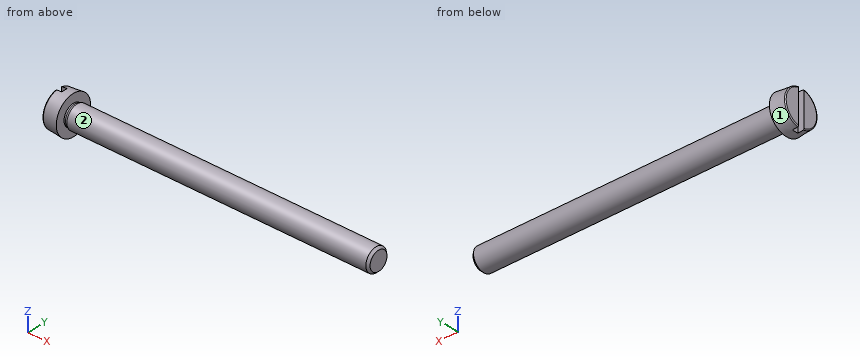
Autodesk Inventor part; units mm, degrees
ref_plane "Work Plane1" through (30.1625, 0, 0) normal (0, 0, -1) x (1, 0, 0)
ref_plane "YZ Plane" through (0, 0, 0) normal (1, 0, 0) x (0, 1, 0)
ref_plane "XZ Plane" through (0, 0, 0) normal (0, 1, 0) x (-1, 0, 0)
sketch "Skizze1" plane through (0, 0, 0) normal (0, 0, 1) x (1, 0, 0)
  line L0 (-3.9, 0) -> (80, 0)
  line L1 (80, 0) -> (80, 3)
  line L2 (80, 3) -> (1, 3)
  line L3 (1, 3) -> (0.3864, 2.7294)
  line L4 (0.3864, 2.7294) -> (0, 2.7294)
  line L5 (0, 2.7294) -> (0, 5)
  line L6 (-20.68, 0) -> (96.78, 0)
  line L7 (0, -1) -> (0, 6)
  line L8 (-3.9, 0) -> (-3.9, 4.6588)
  line L9 (0, 5) -> (-3.9, 4.6588)
  line L10 (1, 3) -> (0, 3) construction
  dimension "d0" = 80
  dimension "d1" = 79
  dimension "d2" = 0.6136
  dimension "d3" = 3.9
  dimension "d4" = 6
  dimension "d5" = 5.4587
  dimension "d9" = 10
  dimension "d10" = 5
revolve "Körper" add sketch "Skizze1" angle 360 about axis through (-3.9, 0, 0) along (1, 0, 0)
sketch "Skizze2" plane through (-3.9, 0, 0) normal (-1, 0, 0) x (0, 0, 1)
  circle A0 centre (0, 0) radius 5
  line L0 (0, 0) -> (0, 4.6588)
  line L1 (-5, 0.8) -> (5, 0.8)
  line L2 (5, 0.8) -> (5, -0.8)
  line L3 (5, -0.8) -> (-5, -0.8)
  line L4 (-5, -0.8) -> (-5, 0.8)
  line L5 (-5, 0) -> (5, 0) construction
  line L6 (0, 0.8) -> (0, -0.8) construction
  dimension "d11" = 1.6
  dimension "d12" = 10
fillet "Rundung1" radius 0.25 1 edges at (-3.9, -4.6588, 0)
extrude "Loch" cut sketch "Skizze2" against normal blind 1.6 contours A0 L3 L1 | L2 L3 A0 | A0 L1 L2 | A0 L4 L1 | L3 L4 A0
thread "Gewinde"
chamfer "Fase1" distance 0.5413 distance2 0.6136 1 edges at (80, -3, 0) measured on face at (80, 0.8631, 0.1984)
ref_plane "Work Plane1" through (30.1625, 0, 0) normal (0, 0, -1) x (1, 0, 0)
equation "\"d11\" = SBR"
equation "\"d12\" = KOD"
equation "\"d14\" = RR"
equation "\"d19\" = STI"
equation "\"d15\" = GEL"
equation "\"d17\" = -0.5 * SPD + 0.5 * GD"
equation "\"d3\" = KOH"
equation "\"d4\" = GD"
equation "\"d5\" = BDM"
equation "\"d9\" = KOD"
equation "\"d10\" = KEWI"
equation "\"GD\" = 6"
equation "\"GEL\" = 38"
equation "\"KOD\" = 10"
equation "\"KOH\" = 3.9"
equation "\"GAL\" = 0.61345 * PTC"
equation "\"SPD\" = 4.91747"
equation "\"BDM\" = 5.45873"
equation "\"GUL\" = 0.61345 * PTC"
equation "\"RR\" = 0.25"
equation "\"SBR\" = 1.6"
equation "\"STI\" = 1.6"
equation "\"KEWI\" = 5deg"
equation "\"PTC\" = 1"
equation "\"THREADDIA\" = 6"
equation "\"TOA\" = 30deg"
equation "\"NND\" = 6"
equation "\"GD1\" = THREADDIA - 1.2269 * PTC"
properties part number "DIN 84 - M6 x 60" material "Stahl, weich"
Source: CAD feature listing. Evaluate the final solid. Frame: model axes, mm. Face numbers are marked on the shaded views. A direction names the side the tool comes from. Give positions to 0.01 mm unless a question says otherwise; leave off trailing zeros. Order: outer loops, then holes, each group sorted by start corner. A loop starts at its lowest first (then second) coordinate and runs counter-clockwise, first axis right, second up.
(1) Section query B-B (x = 51.5). Return the cut outline in (y, z), plus the area to 3 significant figures.
(2) Contact query for flat-ended pins moving along their axis: P1, Ø1.8, axis at x = -3.5, z = 1, coming from the +Y side; P2, Ø1.5, axis at x = 19.5, z = -2.5, coming from the -Y side; P3, Ø5, axis at x = 57, y = 3.5, coming from the -Z side. Output: stop coordinate, or through.
(3) Access query for the marked faces 1 and 2. Directions: +Z, -Z, +X, -X, +Y, -Y. A direction counts if a zero-diameter tool reaches every point of the face in a straight line with its end or side. Return the directions, or none.
(4) Material intervals for line 1 along Z through (x, y) = (46.5, -1.25); line 2 along X through (y, z) = (2.25, -3.75), sorted ascending.
(5) Section query A-A (y = 0). Return the cut outline in (x, z).
Outcome:
1. outline: circle Ø6 at (0, 0)
1. area: 28.3 mm2
2. P1: stops at y = 4.74
2. P2: stops at y = -2.44
2. P3: stops at z = -2.83
3. face 1: -X
3. face 2: +X
4. line 1: z = -2.73 to 2.73
4. line 2: x = -3.9 to 0
5. outline: (-2.3, -4.8) - (0, -5) - (0, -2.73) - (0.39, -2.73) - (1, -3) - (79.39, -3) - (80, -2.46) - (80, 2.46) - (79.39, 3) - (1, 3) - (0.39, 2.73) - (0, 2.73) - (0, 5) - (-2.3, 4.8) - close
